The figure shows three views and two pictorial views of one solid part (mm, origin at its lowest corner). Answer the questions. Coordinates: 2 decimals unless noted, no trailing zeros. Write each loop counter-clockwise with the first axis right and the second up, starting at its lowest first coordinate (ties: lowest second). Pieces come first, ordered by that corner, then holes.
Item 1: Each of these flat-tipped pins is pushed along its axis until it touches: P1, Ø0.9, axis at x = 8.5, y = 1.5, coming from the +Z side; P2, Ø0.9, axis at x = 6.5, y = 2, coming from the -Z side. Where does it stop, or does it pass through?
Item 2: Section A-A (z = 84.42) is taken. Give the vertices of the cut face in (x, y), then the cut area to 3 significant figures.
Item 3: Section C-C (y = 0.65) is taken. Give the vertices of the cut face in (x, z), then the cut area to 3 significant figures.
Item 4: Straight lines are drawn through the part: probe 1 along Z at (x, y) = (7, 2.2); probe 2 along X at (y, z) = (1.45, 79.42); probe 3 along X at (y, z) = (2.55, 87). For each, find the intervals that lie inside material, in ascending order.
Item 5: Section B-B (x = 97) is taken. Give the vertices of the cut face in (y, z).
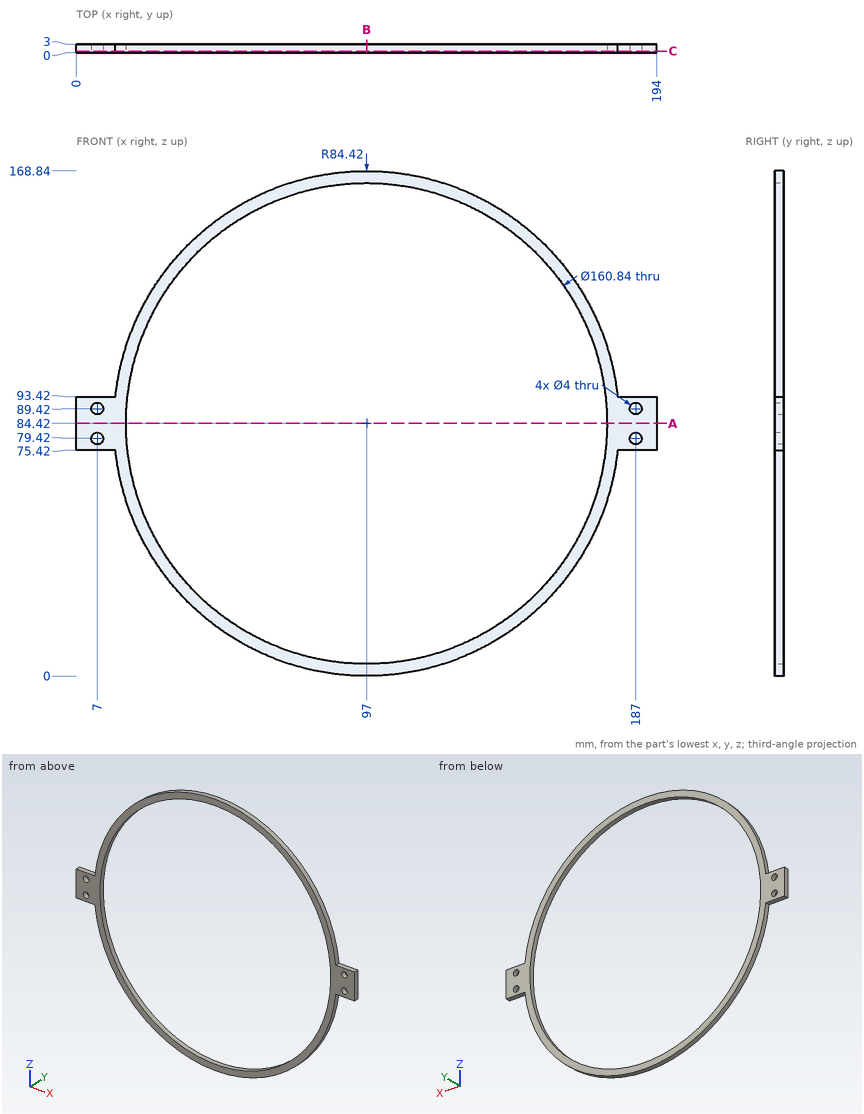
Established:
1. P1: stops at z = 93.42
1. P2: stops at z = 75.42
2. outline: (0, 0) - (16.58, 0) - (16.58, 3) - (0, 3) - close; (177.42, 0) - (194, 0) - (194, 3) - (177.42, 3) - close
2. area: 99.5 mm2
3. outline: (0, 75.42) - (13.06, 75.42) arc R84.42 ccw to (180.94, 75.42) - (194, 75.42) - (194, 93.42) - (180.94, 93.42) arc R84.42 ccw to (13.06, 93.42) - (0, 93.42) - close; hole circle Ø4 at (7, 79.42); hole circle Ø4 at (7, 89.42); hole circle Ø160.84 at (97, 84.42); hole circle Ø4 at (187, 79.42); hole circle Ø4 at (187, 89.42)
3. area: 2,480 mm2
4. probe 1: z = 75.42 to 77.42, 81.42 to 87.42, 91.42 to 93.42
4. probe 2: x = 0 to 5, 9 to 16.74, 177.26 to 185, 189 to 194
4. probe 3: x = 0 to 16.62, 177.38 to 194
5. outline: (0, 0) - (3, 0) - (3, 4) - (0, 4) - close; (0, 164.84) - (3, 164.84) - (3, 168.84) - (0, 168.84) - close
